Build history of the part. All positions in model axes, mm. Face numbers are marked on the shaded views. Round coordinates to 2 decimals unless told otherwise and drop trailing zeros. Write each loop counter-clockwise with the first axis right and the second up, starting at its lowest first coordinate (ties: lowest second). Pieces come first, ordered by that corner, then holes. Notation, with made-up numbers: (-31, -2) - (22, -2) arc R35 cw to (22, 37) - close; hole circle Ø3 at (-9, -13). An arc over 180 degrees is marked (long way). Answer as a JSON object with one key per item and string values. Group by question number.
Item 1: Slice it at D-D, the plane z = 27.5. List the corners of the cut face in (x, y), then the cut area to 3 significant figures.
Item 2: Slice it at C-C, the plane y = 1. List the corners of the cut face in (x, z), then the cut area to 3 significant figures.
Item 3: Flat gauge pins, fed straight in: pin 1 (1 mm diameter, centred on x = -7, y = -2.5, fed in from -Z); pin 2 (0.6 mm diameter, centred on x = -12, y = -1.5, fed in from +Z); pin 3 (3 mm diameter, centred on x = -30.5, y = -1, fed in from +Z); pin 4 (10 mm diameter, centred on x = -22, z = -11.5, fed in from -Y). Where does each tip first touch, or does it go through?
Item 4: Slice it at B-B, the plane z = 0. List the corners of the cut face in (x, y), then the cut area to 3 significant figures.
Item 5: Two-plate mould, pull along Z, no slides. Class the marked faces 1, 2 and 3: +Z half, -Z half, draft (parallel to the pull), parting line (faces both ways), or undercut.
Item 6: Slice it at A-A, the plane x = 0. List the corners of the cut face in (y, z).
Item 7: Probe line 1 (X direction, y = 3, z = 0); line 2 (X direction, y = 3, z = -15.5); line 3 (Y direction, x = 9, z = 19). List the from-to ranges inside material, lowest first. Write a range as from..to.
from build123d import *

# Parameters (mm, degrees)
SKETCH2_W               = 1
SKETCH2_H               = 0.5
SKETCH2_W_2             = 1.3
SKETCH2_H_2             = 0.65
CUT_EXTRUDE2_DEPTH      = 5.15
CUT_EXTRUDE2_DEPTH_BACK = 4.65


with BuildPart() as part:
    # Sketch2 → Revolve1 (revolve)
    with BuildSketch(Plane(origin=(0, 0, 0), x_dir=(0, 0, -1), z_dir=(1, 0, 0))):
        Polygon((-49, 3.65), (-50, 3.65), (-50, -3.65), (-48, -3.65), (-48, -2.15), (-48, -0.15), (-48, 3.65), align=None)
        with Locations((-48.5, 3.9)):
            Rectangle(SKETCH2_W, SKETCH2_H)
        Polygon((-23.6, -0.15), (-48, -0.15), (-48, -2.15), (-20, -2.15), (-20, -0.15), align=None)
        Polygon((-23.6, 2.5), (-23.6, -0.15), (-20, -0.15), (-20, 2.5), (-22.3, 2.5), align=None)
        with Locations((-22.95, 2.825)):
            Rectangle(SKETCH2_W_2, SKETCH2_H_2)
    revolve(axis=Axis((0, 0, 0), (0, 1, 0)))

    # Sketch3 → Cut-Extrude2 (cut, two sides)
    with BuildSketch(Plane(origin=(0, 0, 0), x_dir=(1, 0, 0), z_dir=(0, 1, 0))) as cut_extrude2_sk:
        with BuildLine():
            Line((-182.0491461, -239.559631704), (-30.252223805, -39.809583706))
            Line((-30.252223805, -39.809583706), (-28.980936876, -38.136693234))
            ThreePointArc((-28.980936876, -38.136693234), (-27.221907589, -36.68275573), (-25, -36.1619439))
            Line((-25, -36.1619439), (25, -36.1619439))
            ThreePointArc((25, -36.1619439), (27.2219242, -36.682763969), (28.980959314, -38.13672276))
            Line((28.980959314, -38.13672276), (30.252211397, -39.809593135))
            Line((30.252211397, -39.809593135), (182.047652189, -239.56076697))
            Line((182.047652189, -239.56076697), (182.046087664, -741.32719587))
            Line((182.046087664, -741.32719587), (-182.050710625, -741.326060604))
            Line((-182.050710625, -741.326060604), (-182.0491461, -239.559631704))
        make_face()
    extrude(amount=CUT_EXTRUDE2_DEPTH, mode=Mode.SUBTRACT)
    extrude(cut_extrude2_sk.sketch, amount=-CUT_EXTRUDE2_DEPTH_BACK, mode=Mode.SUBTRACT)


solid = part.part
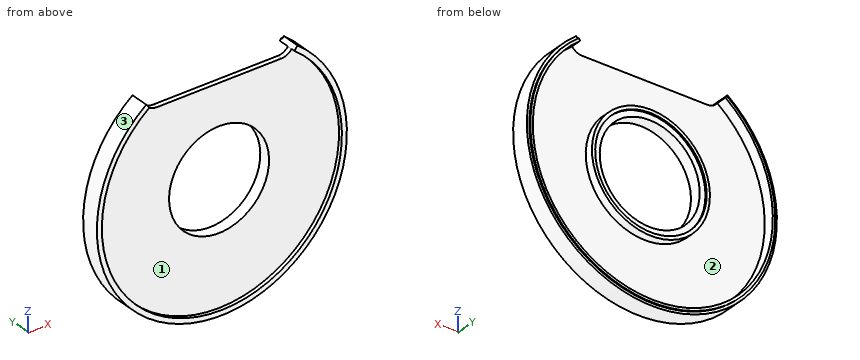
Geometry says:
{
 "1": {"outline": "(-41.76, -3.65) - (-39.34, -3.65) - (-39.34, -2.15) - (39.34, -2.15) - (39.34, -3.65) - (41.76, -3.65) - (41.76, 3.65) - (40.56, 3.65) - (40.56, 4.15) - (39.34, 4.15) - (39.34, -0.15) - (-39.34, -0.15) - (-39.34, 4.15) - (-40.56, 4.15) - (-40.56, 3.65) - (-41.76, 3.65) - close", "area": "194 mm^2"},
 "2": {"outline": "(-30.25, 39.81) arc R50 ccw (long way) to (30.25, 39.81) - (29.04, 38.22) arc R48 cw (long way) to (-29.04, 38.22) - close; circle Ø47.2 at (0, 0); hole circle Ø40 at (0, 0)", "area": "981 mm^2"},
 "3": {"pin 1": "stops at z = -49.58", "pin 2": "stops at z = 36.16", "pin 3": "stops at z = 39.81", "pin 4": "stops at y = -2.15"},
 "4": {"outline": "(-50, -3.65) - (-48, -3.65) - (-48, -2.15) - (-20, -2.15) - (-20, 2.5) - (-22.3, 2.5) - (-22.3, 3.15) - (-23.6, 3.15) - (-23.6, -0.15) - (-48, -0.15) - (-48, 4.15) - (-49, 4.15) - (-49, 3.65) - (-50, 3.65) - close; (20, -2.15) - (48, -2.15) - (48, -3.65) - (50, -3.65) - (50, 3.65) - (49, 3.65) - (49, 4.15) - (48, 4.15) - (48, -0.15) - (23.6, -0.15) - (23.6, 3.15) - (22.3, 3.15) - (22.3, 2.5) - (20, 2.5) - close", "area": "163 mm^2"},
 "5": {"face 1": "undercut", "face 2": "undercut", "face 3": "parting line"},
 "6": {"outline": "(-3.65, -50) - (3.65, -50) - (3.65, -49) - (4.15, -49) - (4.15, -48) - (-0.15, -48) - (-0.15, -23.6) - (3.15, -23.6) - (3.15, -22.3) - (2.5, -22.3) - (2.5, -20) - (-2.15, -20) - (-2.15, -48) - (-3.65, -48) - close; (-2.15, 20) - (2.5, 20) - (2.5, 22.3) - (3.15, 22.3) - (3.15, 23.6) - (-0.15, 23.6) - (-0.15, 36.16) - (-2.15, 36.16) - close"},
 "7": {"line 1": "x = -50..-48, -23.6..-22.3, 22.3..23.6, 48..50", "line 2": "x = -47.54..-45.43, -17.8..-16.03, 16.03..17.8, 45.43..47.54", "line 3": "y = -2.15..2.5"}
}
